Answer from the drawing. Dimensions are ordinates in mm from the lowest x, y and z of the part. A direction names the side the tool comes from. Round coordinates to 2 decimals unless told otherwise and drop trailing zeros. Loops run counter-clockwise (first coordinate to the right, second up) from the corner with the lowest first, then second, coordinate; pieces in that order, holes last. Notation, with made-up numbers: M -39.5,25.5 L 5.5,25.5 A26 ccw 5.5,43.5 Z; hole C -34,10 d4. An arc over 180 degrees is marked long. Answer as a JSON object with one key per item and string values.
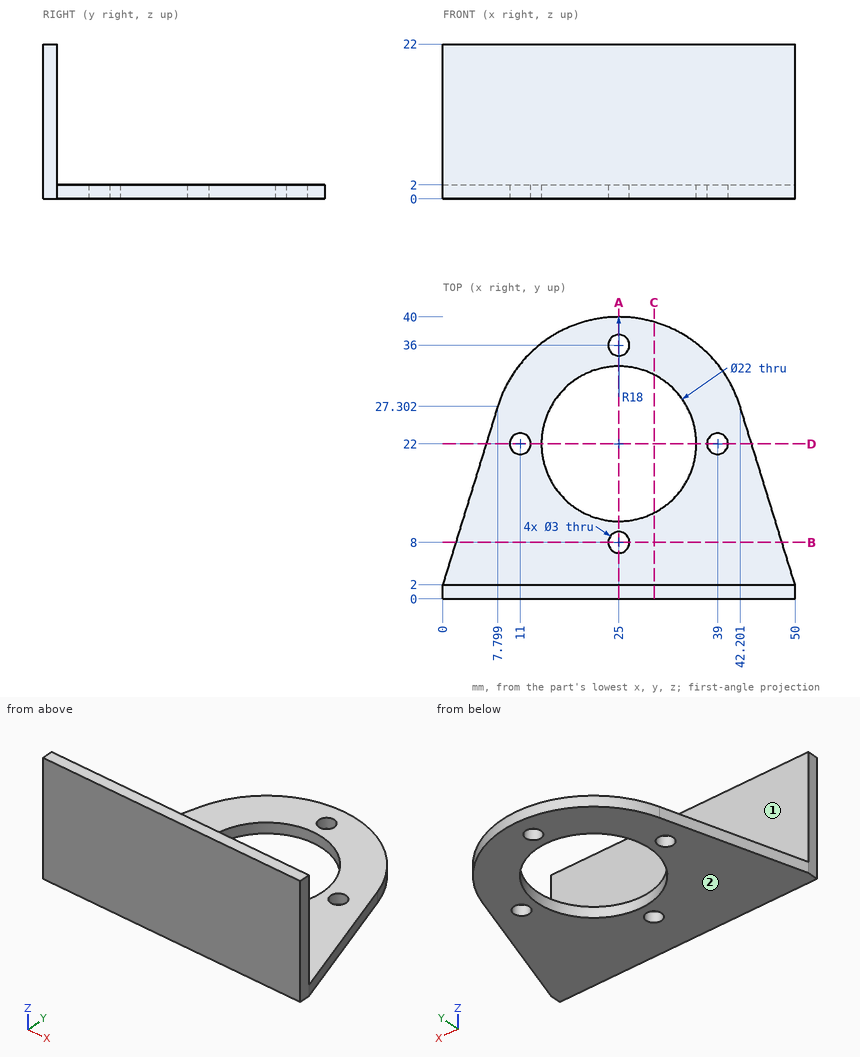
Item 1: The part is cut by section A-A (x = 25). Give the vertices of the cut face in (y, z).
Values follow:
{"outline": "M 0,0 L 6.5,0 L 6.5,2 L 2,2 L 2,22 L 0,22 Z; M 9.5,0 L 11,0 L 11,2 L 9.5,2 Z; M 33,0 L 34.5,0 L 34.5,2 L 33,2 Z; M 37.5,0 L 40,0 L 40,2 L 37.5,2 Z"}
Item 2: The part is cut by section D-D (y = 22). Give the vertices of the cut face in (x, z) (1 decimal).
Values follow:
{"outline": "M 6.2,0 L 9.5,0 L 9.5,2 L 6.2,2 Z; M 12.5,0 L 14,0 L 14,2 L 12.5,2 Z; M 36,0 L 37.5,0 L 37.5,2 L 36,2 Z; M 40.5,0 L 43.8,0 L 43.8,2 L 40.5,2 Z"}
Item 3: The part is cut by section B-B (y = 8). Give the vertices of the cut face in (x, z).
Values follow:
{"outline": "M 1.85,0 L 23.5,0 L 23.5,2 L 1.85,2 Z; M 26.5,0 L 48.15,0 L 48.15,2 L 26.5,2 Z"}
Item 4: Which of the six approach directions +Z, -Z, +X, -X, +Y, -Y give full straight-line access (tool end or side, diameter ignored) to the marked faces 1 and 2?
Values follow:
{"face 1": "+Z, +X, -X, +Y", "face 2": "-Z, +X, -X, +Y, -Y"}
Item 5: Straight lines are drawn through the part: line 1 (Y direction, x = 25, z = 1); line 2 (Z direction, x = 9, y = 25). For each, find the intervals that lie inside material, in ascending order.
Values follow:
{"line 1": "0 to 6.5, 9.5 to 11, 33 to 34.5, 37.5 to 40", "line 2": "0 to 2"}
Item 6: The part is cut by section C-C (x = 30). Give the vertices of the cut face in (y, z).
Values follow:
{"outline": "M 0,0 L 12.2,0 L 12.2,2 L 2,2 L 2,22 L 0,22 Z; M 31.8,0 L 39.29,0 L 39.29,2 L 31.8,2 Z"}
Item 7: Flat-ended cylindrical pins translate along their axes: P1, Ø10, axis at x = 23.5, y = 9, coming from the -Z side; P2, Ø8, axis at x = 17.5, z = 4.5, coming from the +Y side; P3, Ø8, axis at x = 24, y = 12, coming from the +Z side; P4, Ø12, axis at y = 26.5, z = 2.5, coming from the -X side. Find the tip coordinate at first contact, or state that the pin passes through.
Values follow:
{"P1": "z = 0", "P2": "y = 39.46", "P3": "z = 2", "P4": "x = 5.71"}
